Input: part model. Units: mm. Frame: model coordinates. Face numbers are marked on the shaded views. Coordinates: 2 decimals unless noted, no trailing zeros. Order: outer loops, then holes, each group sorted by start corner. A loop starts at its lowest first (then second) coordinate and runs counter-clockwise, first axis right, second up.
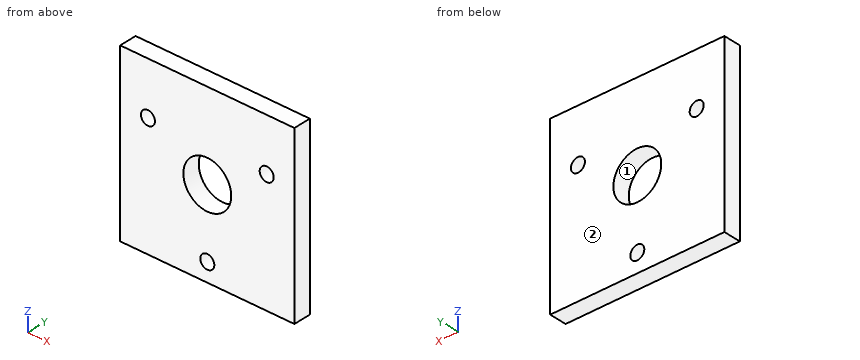
from build123d import *

# Parameters (mm, degrees)
SKETCH1_W           = 63.5
SKETCH1_H           = 63.5
SKETCH1_R           = 2.5527
SKETCH1_R_2         = 8.73125
BOSS_EXTRUDE1_DEPTH = 6.35


with BuildPart() as part:
    # Sketch1 → Boss-Extrude1 (new body)
    with BuildSketch(Plane(origin=(0, 0, 0), x_dir=(1, 0, 0), z_dir=(0, 1, 0))):
        Rectangle(SKETCH1_W, SKETCH1_H)
        with Locations((0, 25)):
            Circle(SKETCH1_R, mode=Mode.SUBTRACT)
        Circle(SKETCH1_R_2, mode=Mode.SUBTRACT)
        with Locations((21.650635095, -12.5)):
            Circle(SKETCH1_R, mode=Mode.SUBTRACT)
        with Locations((-21.650635095, -12.5)):
            Circle(SKETCH1_R, mode=Mode.SUBTRACT)
    extrude(amount=BOSS_EXTRUDE1_DEPTH)


solid = part.part
Item 1: Cut plane A-A on x = 0. Return loops of the section in (y, z), then the cut area to 3 significant figures.
Response values:
outline: (0, -31.75) - (6.35, -31.75) - (6.35, -27.55) - (0, -27.55) - close; (0, -22.45) - (6.35, -22.45) - (6.35, -8.73) - (0, -8.73) - close; (0, 8.73) - (6.35, 8.73) - (6.35, 31.75) - (0, 31.75) - close
area: 260 mm2
Item 2: Cut plane C-C on z = 0. Return loops of the section in (x, y).
Response values:
outline: (-31.75, 0) - (-8.73, 0) - (-8.73, 6.35) - (-31.75, 6.35) - close; (8.73, 0) - (31.75, 0) - (31.75, 6.35) - (8.73, 6.35) - close
Item 3: Ray query, probe 1 along X at (y, z) = (1.5, 12.5); probe 2 along Z at (x, y) = (0, 3.75); probe 3 along X at (y, z) = (5.25, 0). Return the intervals inside material, ascending.
Response values:
probe 1: x = -31.75 to -24.2, -19.1 to 19.1, 24.2 to 31.75
probe 2: z = -31.75 to -27.55, -22.45 to -8.73, 8.73 to 31.75
probe 3: x = -31.75 to -8.73, 8.73 to 31.75
Item 4: Cut plane D-D on y = 3.25. Return loops of the section in (x, z).
Response values:
outline: (-31.75, -31.75) - (31.75, -31.75) - (31.75, 31.75) - (-31.75, 31.75) - close; hole circle Ø5.11 at (-21.65, 12.5); hole circle Ø17.46 at (0, 0); hole circle Ø5.11 at (0, -25); hole circle Ø5.11 at (21.65, 12.5)
Item 5: Draft query along X for the marked faces 1 and 2. Return one class per face: pulls with the +X half, pulls with the -X half, needs draft (parallel to the pull), parting line crosses it, or undercut.
Response values:
face 1: undercut
face 2: needs draft
Item 6: Pin query (flat end, axial travel): pin 1 Ø4.5 at (x, z) = (21.65, 12.5) entering from -Y. Return the tip coordinate at first contact, or that it passes through.
Response values:
pin 1: passes through
Item 7: Cut plane B-B on z = 12.5. Return loops of the section in (x, y).
Response values:
outline: (-31.75, 0) - (-24.2, 0) - (-24.2, 6.35) - (-31.75, 6.35) - close; (-19.1, 0) - (19.1, 0) - (19.1, 6.35) - (-19.1, 6.35) - close; (24.2, 0) - (31.75, 0) - (31.75, 6.35) - (24.2, 6.35) - close
